```python
from build123d import *

# Parameters (mm, degrees)
CROQUIS1_W              = 350
CROQUIS1_H              = 60
SALIENTE_EXTRUIR1_DEPTH = 6
CROQUIS2_R              = 6
CROQUIS2_R_2            = 1.25
CORTAR_EXTRUIR1_DEPTH   = 7
CORTAR_EXTRUIR4_DEPTH   = 1.5
CROQUIS4_R              = 4
CORTAR_EXTRUIR5_DEPTH   = 7


with BuildPart() as part:
    # Croquis1 → Saliente-Extruir1 (new body)
    with BuildSketch(Plane.XY):
        with Locations((-175, -30)):
            Rectangle(CROQUIS1_W, CROQUIS1_H)
    extrude(amount=SALIENTE_EXTRUIR1_DEPTH)

    # Croquis2 → Cortar-Extruir1 (cut, through all)
    with BuildSketch(Plane.XY.offset(6)):
        with Locations((-327.5, -22.5)):
            Circle(CROQUIS2_R)
        with Locations((-22.5, -22.5)):
            Circle(CROQUIS2_R)
        with Locations((-314.595301243, -9.595301243)):
            Circle(CROQUIS2_R_2)
        with Locations((-340.404698757, -35.404698757)):
            Circle(CROQUIS2_R_2)
        with Locations((-35.404698757, -9.595301243)):
            Circle(CROQUIS2_R_2)
        with Locations((-9.595301243, -35.404698757)):
            Circle(CROQUIS2_R_2)
    extrude(amount=-CORTAR_EXTRUIR1_DEPTH, mode=Mode.SUBTRACT)

    # Croquis3 → Cortar-Extruir4 (cut)
    with BuildSketch(Plane.XY):
        with BuildLine():
            Line((-98, 0), (-58, 0))
            Line((-58, 0), (-58, -36))
            ThreePointArc((-58, -36), (-59.171572875, -38.828427125), (-62, -40))
            Line((-62, -40), (-94, -40))
            ThreePointArc((-94, -40), (-96.828427125, -38.828427125), (-98, -36))
            Line((-98, -36), (-98, 0))
        make_face()
        with BuildLine():
            Line((-292, 0), (-252, 0))
            Line((-252, 0), (-252, -36))
            ThreePointArc((-252, -36), (-253.171572875, -38.828427125), (-256, -40))
            Line((-256, -40), (-288, -40))
            ThreePointArc((-288, -40), (-290.828427125, -38.828427125), (-292, -36))
            Line((-292, -36), (-292, 0))
        make_face()
    extrude(amount=CORTAR_EXTRUIR4_DEPTH, mode=Mode.SUBTRACT)

    # Croquis4 → Cortar-Extruir5 (cut, through all)
    with BuildSketch(Plane.XY.offset(6)):
        with Locations((-272, -20)):
            Circle(CROQUIS4_R)
        with Locations((-78, -20)):
            Circle(CROQUIS4_R)
    extrude(amount=-CORTAR_EXTRUIR5_DEPTH, mode=Mode.SUBTRACT)


solid = part.part
```
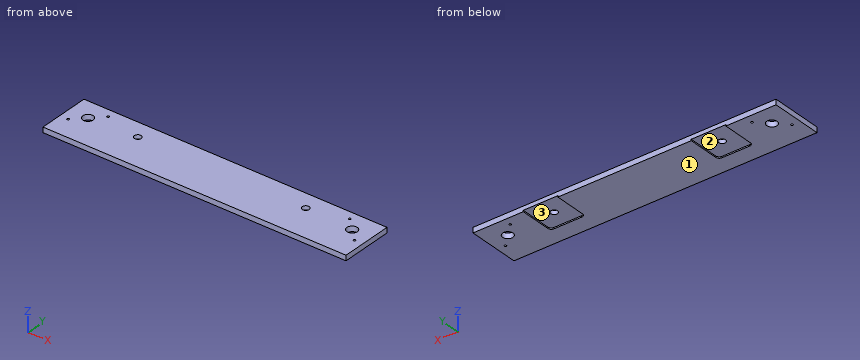
The model under review builds one solid part; all positions refer to its coordinate system, in mm. Face numbers are marked on the shaded views. Round coordinates to 2 decimals unless told otherwise and drop trailing zeros. Loops run counter-clockwise (first coordinate to the right, second up) from the corner with the lowest first, then second, coordinate; pieces in that order, holes last. Notation, with made-up numbers: (7, -20.5) -> (32, -20.5) arc R10 ccw to (32, -2.5) -> close; hole circle Ø10 at (27, 70.5). An arc over 180 degrees is marked (long way). Answer in a Markdown table with one row per item.
1) Draft analysis for pull direction X (two halves, no side actions). For the marked faces 1, 2 and 3, state which applies: pulls with the +X half, pulls with the -X half, needs draft (parallel to the pull), parting line crosses it, or undercut.
Taken from the geometry:
| item | result |
|---|---|
| face 1 | needs draft |
| face 2 | undercut |
| face 3 | undercut |
2) Consider section A-A, the plane x = -327.5. Write out the cut boundary in (y, z), plus the area to 3 significant figures.
Taken from the geometry:
| item | result |
|---|---|
| outline | (-60, 0) -> (-28.5, 0) -> (-28.5, 6) -> (-60, 6) -> close; (-16.5, 0) -> (0, 0) -> (0, 6) -> (-16.5, 6) -> close |
| area | 288 mm² |
3) Consider section B-B, the plane x = -78. Write out the cut boundary in (y, z), plus the area to 3 significant figures.
Taken from the geometry:
| item | result |
|---|---|
| outline | (-60, 0) -> (-40, 0) -> (-40, 1.5) -> (-24, 1.5) -> (-24, 6) -> (-60, 6) -> close; (-16, 1.5) -> (0, 1.5) -> (0, 6) -> (-16, 6) -> close |
| area | 264 mm² |
4) For pin 1 Ø3 at (x, y) = (-314.6, -9.6) entering from +Z; pin 2 Ø2 at (x, y) = (-340.4, -35.4) entering from +Z; pin 3 Ø20 at (x, y) = (-79.5, -14.5) entering from -Z, all flat-tipped, find the tip position at first contact; note any pin that passes through.
Taken from the geometry:
| item | result |
|---|---|
| pin 1 | stops at z = 6 |
| pin 2 | passes through |
| pin 3 | stops at z = 1.5 |
5) Consider section C-C, the plane z = 2.75. Count the separate pieces of the cut face and the enclosed holes in it, plus the area to 3 significant figures.
Taken from the geometry:
| item | result |
|---|---|
| separate pieces | 1 |
| enclosed holes | 8 |
| area | 20,700 mm² |
6) Wall thickness on line 1 along X through (y, z) = (-3.5, 0.85); line 2 along Y through (x, z) = (-327.5, 4.35); line 3 along X through (y, z) = (-36.5, 4.5): over which ranges is each line inside the solid? List them lowest first.
Taken from the geometry:
| item | result |
|---|---|
| line 1 | x = -350 to -292, -252 to -98, -58 to 0 |
| line 2 | y = -60 to -28.5, -16.5 to 0 |
| line 3 | x = -350 to -341.01, -339.8 to -10.2, -8.99 to 0 |
